Design review of the part built by this model. Coordinates are the model's own, in mm. A direction names the side the tool comes from. Coordinates: 2 decimals unless noted, no trailing zeros. Write each loop counter-clockwise with the first axis right and the second up, starting at its lowest first coordinate (ties: lowest second). Pieces come first, ordered by that corner, then holes. Notation, with made-up numbers: (22.25, 71) -> (55.25, 71) arc R12 cw to (55.25, 80) -> close; hole circle Ø5 at (-24.5, 67.5). An arc over 180 degrees is marked (long way). Answer in a Markdown table with one row per item. Add a question column.
Item 1: For faces 1 (the face through (-10, 0, 39.624)), 2 (the face through (-1, -3.175, -1)), 3 (the face through (-9, 0, -39.624)), list the 3-axis set-ups (+Z, -Z, +X, -X, +Y, -Y) from which the entire face can be reached by the end or side of a thin tool; tool diameter is ignored.
Item 2: Take a section at D-D, the plane z = 36.5. Write out the cut boundary in (x, y) (3 decimals), and give its area (3 significant figures).
Item 3: Take a section at B-B, the plane z = 6. Write out the cut boundary in (x, y) (3 decimals).
Item 4: Clearance check with flat-ended pins moving along their axes: P1, Ø1, axis at y = 1.5, z = -33.5, coming from the +X side (3 decimals); P2, Ø2.5, axis at x = 14.68, z = -34.21, coming from the +Y side; P3, Ø3, axis at y = 0, z = 25.5, coming from the -X side (3 decimals); P4, Ø3, axis at x = -20.5, y = -0.5, coming from the -Z side. State where each tip first meets the part, or that it passes through.
Item 5: To check wall thickness, follow line 1 (X direction, y = 0.5, z = 5) (3 decimals); line 2 (X direction, y = 2, z = 9) (3 decimals); line 3 (X direction, y = 0.5, z = 59.5) (3 decimals). State the ranges of each line that lie inside material, in increasing order.
Item 6: Take a section at C-C, the plane y = -0.5. Give the number of separate pieces and of enclosed holes in the cut face, and give its area (3 significant figures).
Item 7: Draft analysis for pull direction Z (two halves, no side actions). For faces 4 (the face through (54, 0, -14.224)), 5 (the face through (-64, 0, 14.224)), 6 (the face through (-80.07, -0.04, -0.67)), state which applies: released by +Z, released by -Z, zero draft, split by the parting line, or undercut.
Item 8: Take a section at A-A, the plane x = 31.75. Write out the cut boundary in (y, z) (3 decimals), and give its area (3 significant figures).
from build123d import *

# Parameters (mm, degrees)
BOSS_EXTRUDE1_DEPTH        = 3.175
CUT_EXTRUDE2_START         = 3.175
SKETCH2_R                  = 5.1562
CUT_EXTRUDE2_DEPTH         = 111.817820597
F_10_24_TAPPED_HOLE1_D     = 3.9624
F_10_24_TAPPED_HOLE1_DEPTH = 6.35
F_10_24_TAPPED_HOLE1_TIP   = 1.190425058


with BuildPart() as part:
    # Sketch1 → Boss-Extrude1 (new, symmetric)
    with BuildSketch(Plane(origin=(0, 0, 0), x_dir=(1, 0, 0), z_dir=(0, 1, 0))):
        Polygon((-85.725, -14.224), (-41.275, -14.224), (-41.275, -39.624), (22.225, -39.624), (22.225, -65.024), (85.725, -65.024), (85.725, 14.224), (22.225, 14.224), (22.225, 39.624), (-41.275, 39.624), (-41.275, 65.024), (-85.725, 65.024), align=None)
    extrude(amount=BOSS_EXTRUDE1_DEPTH, both=True)

    # Sketch2 → Cut-Extrude2 (cut, through all)
    with BuildSketch(Plane(origin=(0, 0, 0), x_dir=(1, 0, 0), z_dir=(0, 1, 0)).offset(CUT_EXTRUDE2_START)):
        with Locations(Location((-31.75, -4.826, 0), (0, 0, 270))):
            Circle(SKETCH2_R)
        with Locations(Location((31.75, -4.826, 0), (0, 0, 270))):
            Circle(SKETCH2_R)
    extrude(amount=-CUT_EXTRUDE2_DEPTH, mode=Mode.SUBTRACT)

    # #10-24 Tapped Hole1
    with Locations(Plane(origin=(0, 3.175, 0), x_dir=(1, 0, 0), z_dir=(0, 1, 0))):
        with Locations((-78.1812, 0.0762), (-48.8188, 59.6138), (-14.6812, -25.3238), (14.6812, 34.2138), (48.8188, -50.7238), (78.1812, 8.8138)):
            Hole(F_10_24_TAPPED_HOLE1_D / 2, depth=F_10_24_TAPPED_HOLE1_DEPTH)
            with Locations((0, 0, -(F_10_24_TAPPED_HOLE1_DEPTH + F_10_24_TAPPED_HOLE1_TIP / 2))):  # 118° drill point
                Cone(0, F_10_24_TAPPED_HOLE1_D / 2, F_10_24_TAPPED_HOLE1_TIP, mode=Mode.SUBTRACT)


solid = part.part
Answers:
| question | item | result |
|---|---|---|
| 1 | face 1 | +Z, -X, +Y, -Y |
| 1 | face 2 | +Z, -Z, +X, -X, -Y |
| 1 | face 3 | -Z, +X, +Y, -Y |
| 2 | outline | (-41.275, -3.175) -> (85.725, -3.175) -> (85.725, 3.175) -> (-41.275, 3.175) -> close |
| 2 | area | 806 mm^2 |
| 3 | outline | (-85.725, -3.175) -> (-36.771, -3.175) -> (-36.771, 3.175) -> (-85.725, 3.175) -> close; (-26.729, -3.175) -> (26.729, -3.175) -> (26.729, 3.175) -> (-26.729, 3.175) -> close; (36.771, -3.175) -> (85.725, -3.175) -> (85.725, 3.175) -> (36.771, 3.175) -> close |
| 4 | P1 | stops at x = 22.225 |
| 4 | P2 | passes through |
| 4 | P3 | stops at x = -41.275 |
| 4 | P4 | stops at z = -39.62 |
| 5 | line 1 | x = -85.725 to -36.903, -26.597 to 26.597, 36.903 to 85.725 |
| 5 | line 2 | x = -85.725 to -34.777, -28.723 to 28.723, 34.777 to 85.725 |
| 5 | line 3 | x = 22.225 to 85.725 |
| 6 | separate pieces | 1 |
| 6 | enclosed holes | 8 |
| 6 | area | 13,300 mm^2 |
| 7 | face 4 | released by -Z |
| 7 | face 5 | released by +Z |
| 7 | face 6 | undercut |
| 8 | outline | (-3.175, -14.224) -> (3.175, -14.224) -> (3.175, -0.33) -> (-3.175, -0.33) -> close; (-3.175, 9.982) -> (3.175, 9.982) -> (3.175, 65.024) -> (-3.175, 65.024) -> close |
| 8 | area | 438 mm^2 |
